Geometry: final body of the model. Coordinates: model frame, mm. Face numbers are marked on the shaded views. A direction names the side the tool comes from. Coordinates: 2 decimals unless noted, no trailing zeros. Order: outer loops, then holes, each group sorted by start corner. A loop starts at its lowest first (then second) coordinate and runs counter-clockwise, first axis right, second up. Notation, with made-up numbers: (-31, 39.5) -> (8, 39.5) arc R22 cw to (8, 48.5) -> close; hole circle Ø1 at (59, 24.25). An arc over 180 degrees is marked (long way). Answer in a Markdown table with one row per item. Add a question column.
1) Section query B-B on y = 32.5. Return the cut outline in (x, z), then the cut area to 3 significant figures.
2) Section query A-A on x = 18. Return the cut outline in (y, z), then the cut area to 4 significant figures.
3) Pull-direction query (X, two-part tool) for the marked faces 4, 5, 6 and 7; classes: +X half, -X half, draft (parallel to the pull), parting line (faces both ways), or undercut.
4) Contact query for flat-ended pins moving along their axis: P1, Ø3, axis at y = 32.5, z = 5, coming from the -X side; P2, Ø2, axis at x = -18, z = 5, coming from the +Y side. Output: stop coordinate, or through.
5) Set-up query: the marked faces 1, 2 and 3. Return all of +Z, -Z, +X, -X, +Y, -Y with unobstructed straight access to the full face (end or side cutting, diameter ignored); none if empty.
6) Section query C-C on z = 8.5. Return the cut outline in (x, y).
7) Section query D-D on x = -10. Return the cut outline in (y, z).
8) Ray query, line 1 (X direction, y = -39.55, z = 5); line 2 (X direction, y = 34.5, z = 5.5); line 3 (Z direction, x = 18, y = -40.85). Return the intervals inside material, ascending. Write a range as from..to.
```python
from build123d import *

# Parameters (mm, degrees)
SKETCH_1_W      = 46
SKETCH_1_H      = 20
EXTRUDE_1_DEPTH = 10
FILLET_1_R      = 3
M3X0_51_D       = 2.5
M3X0_51_DEPTH   = 5
M3X0_52_D       = 2.5


with BuildPart() as part:
    # Эскиз1 → Бобышка-Вытянуть1 (new body)
    with BuildSketch(Plane.XY):
        Polygon((-28, 42.5), (-23, 42.5), (-23, -7.5), (23, -7.5), (23, 42.5), (28, 42.5), (28, -42.5), (-28, -42.5), align=None)
        with Locations((0, -27.5)):
            Rectangle(SKETCH_1_W, SKETCH_1_H, mode=Mode.SUBTRACT)
    extrude(amount=EXTRUDE_1_DEPTH)

    # Скругление1
    fillet_1_edges = [part.edges().sort_by_distance(p)[0] for p in [
        (-23, 42.5, 5),
        (-23, -7.5, 5),
        (23, -7.5, 5),
        (23, 42.5, 5),
        (23, -37.5, 5),
        (23, -17.5, 5),
        (-23, -17.5, 5),
        (-23, -37.5, 5),
    ]]
    fillet(fillet_1_edges, radius=FILLET_1_R)

    # Отверстие обработанное метчиком M3x0.51
    with Locations(Plane(origin=(0, -42.5, 0), x_dir=(-1, 0, 0), z_dir=(0, -1, 0))):
        with Locations((18, -5), (-18, -5)):
            Hole(M3X0_51_D / 2, depth=M3X0_51_DEPTH)

    # Отверстие обработанное метчиком M3x0.52 (through all)
    with Locations(Plane(origin=(28, 0, 0), x_dir=(0, 0, -1), z_dir=(1, 0, 0))):
        with Locations((-5, 32.5), (-5, -27.5)):
            Hole(M3X0_52_D / 2)


solid = part.part
```
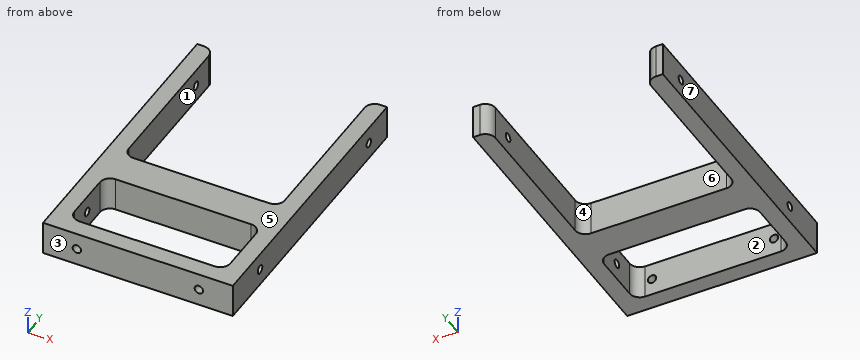
Result:
| question | item | result |
|---|---|---|
| 1 | outline | (-28, 0) -> (-23, 0) -> (-23, 3.75) -> (-28, 3.75) -> close; (-28, 6.25) -> (-23, 6.25) -> (-23, 10) -> (-28, 10) -> close; (23, 0) -> (28, 0) -> (28, 3.75) -> (23, 3.75) -> close; (23, 6.25) -> (28, 6.25) -> (28, 10) -> (23, 10) -> close |
| 1 | area | 75.0 mm2 |
| 2 | outline | (-42.5, 0) -> (-37.5, 0) -> (-37.5, 3.75) -> (-42.5, 3.75) -> close; (-42.5, 6.25) -> (-37.5, 6.25) -> (-37.5, 10) -> (-42.5, 10) -> close; (-17.5, 0) -> (-7.5, 0) -> (-7.5, 10) -> (-17.5, 10) -> close |
| 2 | area | 137.5 mm2 |
| 3 | face 4 | undercut |
| 3 | face 5 | draft |
| 3 | face 6 | undercut |
| 3 | face 7 | -X half |
| 4 | P1 | x = -28 |
| 4 | P2 | y = -7.5 |
| 5 | face 1 | +Z, -Z, +Y |
| 5 | face 2 | +Z, -Z |
| 5 | face 3 | +Z, -Z, +X, -X, -Y |
| 6 | outline | (-28, -42.5) -> (28, -42.5) -> (28, 42.5) -> (26, 42.5) arc R3 ccw to (23, 39.5) -> (23, -4.5) arc R3 cw to (20, -7.5) -> (-20, -7.5) arc R3 cw to (-23, -4.5) -> (-23, 39.5) arc R3 ccw to (-26, 42.5) -> (-28, 42.5) -> close; hole (-23, -34.5) arc R3 ccw to (-20, -37.5) -> (20, -37.5) arc R3 ccw to (23, -34.5) -> (23, -20.5) arc R3 ccw to (20, -17.5) -> (-20, -17.5) arc R3 ccw to (-23, -20.5) -> close |
| 7 | outline | (-42.5, 0) -> (-37.5, 0) -> (-37.5, 10) -> (-42.5, 10) -> close; (-17.5, 0) -> (-7.5, 0) -> (-7.5, 10) -> (-17.5, 10) -> close |
| 8 | line 1 | -28..-19.25, -16.75..16.75, 19.25..28 |
| 8 | line 2 | -28..-23, 23..28 |
| 8 | line 3 | 0..3.75, 6.25..10 |
